from build123d import *

# Parameters (mm, degrees)
SKETCH1_R           = 17.5
BOSS_EXTRUDE1_DEPTH = 14
SKETCH2_R           = 1.5
BOSS_EXTRUDE2_DEPTH = 1
SKETCH3_R           = 5
BOSS_EXTRUDE3_DEPTH = 1.5
SKETCH4_R           = 1.5
BOSS_EXTRUDE4_DEPTH = 11
SKETCH5_R           = 3
BOSS_EXTRUDE5_DEPTH = 0.5
SKETCH6_R           = 1.5
BOSS_EXTRUDE6_DEPTH = 0.1
FILLET1_R           = 0.5
SKETCH7_W           = 7
SKETCH7_H           = 7.8
CUT_EXTRUDE3_DEPTH  = 2


with BuildPart() as part:
    # Sketch1 → Boss-Extrude1 (new body)
    with BuildSketch(Plane(origin=(0, 0, 0), x_dir=(1, 0, 0), z_dir=(0, 1, 0))):
        Circle(SKETCH1_R)
    extrude(amount=BOSS_EXTRUDE1_DEPTH)

    # Sketch2 → Boss-Extrude2 (add)
    with BuildSketch(Plane.XZ):
        with BuildLine():
            Line((14.671631406, 18.344732976), (-0.891940662, 17.553925067))
            ThreePointArc((-0.891940662, 17.553925067), (-12.428512449, 12.428512449), (-17.553925067, 0.891940662))
            Line((-17.553925067, 0.891940662), (-18.344732976, -14.671631406))
            ThreePointArc((-18.344732976, -14.671631406), (-17.324116139, -17.324116139), (-14.671631406, -18.344732976))
            Line((-14.671631406, -18.344732976), (0.891940662, -17.553925067))
            ThreePointArc((0.891940662, -17.553925067), (12.428512449, -12.428512449), (17.553925067, -0.891940662))
            Line((17.553925067, -0.891940662), (18.344732976, 14.671631406))
            ThreePointArc((18.344732976, 14.671631406), (17.324116139, 17.324116139), (14.671631406, 18.344732976))
        make_face()
        with Locations((14.849242405, 14.849242405)):
            Circle(SKETCH2_R, mode=Mode.SUBTRACT)
        with Locations((-14.849242405, -14.849242405)):
            Circle(SKETCH2_R, mode=Mode.SUBTRACT)
    extrude(amount=BOSS_EXTRUDE2_DEPTH)

    # Sketch3 → Boss-Extrude3 (add)
    with BuildSketch(Plane.XZ.offset(1)):
        Circle(SKETCH3_R)
    extrude(amount=BOSS_EXTRUDE3_DEPTH)

    # Sketch4 → Boss-Extrude4 (add)
    with BuildSketch(Plane.XZ.offset(2.5)):
        Circle(SKETCH4_R)
    extrude(amount=BOSS_EXTRUDE4_DEPTH)

    # Sketch5 → Boss-Extrude5 (add)
    with BuildSketch(Plane(origin=(0, 14, 0), x_dir=(1, 0, 0), z_dir=(0, 1, 0))):
        Circle(SKETCH5_R)
    extrude(amount=BOSS_EXTRUDE5_DEPTH)

    # Sketch6 → Boss-Extrude6 (add)
    with BuildSketch(Plane(origin=(0, 14.5, 0), x_dir=(1, 0, 0), z_dir=(0, 1, 0))):
        Circle(SKETCH6_R)
    extrude(amount=BOSS_EXTRUDE6_DEPTH)

    # Fillet1
    fillet1_edges = [part.edges().sort_by_distance(p)[0] for p in [
        (-17.5, 14, 0),
    ]]
    fillet(fillet1_edges, radius=FILLET1_R)

    # Sketch7 → Cut-Extrude3 (cut)
    with BuildSketch(Plane.XY.offset(17.5)):
        with Locations((0, 6.75)):
            Rectangle(SKETCH7_W, SKETCH7_H)
    extrude(amount=-CUT_EXTRUDE3_DEPTH, mode=Mode.SUBTRACT)


solid = part.part
Geometry: final body of the model. Coordinates: model frame, mm. A direction names the side the tool comes from. Give positions to 0.01 mm unless a question says otherwise; leave off trailing zeros. Loops run counter-clockwise (first coordinate to the right, second up) from the corner with the lowest first, then second, coordinate; pieces in that order, holes last. Notation, with made-up numbers: M 32.25,89.25 L 43.25,89.25 A25 cw 43.25,115.25 Z; hole C -3,-16.75 d2. An arc over 180 degrees is marked long. Put each result on its own line as item: value. Start each with the question number.
1) Ray query, line 1 along Y through (x, z) = (-12.5, -13.5); line 2 along Y through (x, z) = (14, 6); line 3 along X through (y, z) = (6.5, -7.5). Return the intervals inside material, ascending.
2) Access query for faces 1 (the flat face through (-3.5, 7, 16)), 2 (the cylindrical face through (12.3, -0.493, -12.556)), 3 (the cylindrical face through (-1.5, -7.92, 0.07)). Directions: +Z, -Z, +X, -X, +Y, -Y. A direction counts if a zero-diameter tool reaches every point of the face in a straight line with its end or side. Return the directions, or none.
3) Cut plane C-C (z = 0). Output: boundary loops of the cut face in (x, y).
4) Contact query for flat-ended pins moving along their axis: pin 1 (10 mm diameter, centred on x = 3, z = -7, fed in from +Y); pin 2 (1.8 mm diameter, centred on y = 8.5, z = 16.5, fed in from +X); pin 3 (5 mm diameter, centred on x = -14.85, z = -14.85, fed in from +Y); pin 4 (12 mm diameter, centred on x = 11.5, y = -8, fed in from -Z) (3 decimals). Output: stop coordinate, or through.
5) Cut plane B-B (y = 6.75). Output: boundary loops of the cut face in (x, z), then the cut area to 3 significant figures.
6) Pull-direction query (Y, two-part tool) for faces 4 (the cylindrical face through (-14.2, -0.5, -16.2)), 5 (the flat face through (0, -13.5, 0)), 6 (the flat face through (3.5, 7, 16)); classes: pulls with the +Y half, pulls with the -Y half, needs draft (parallel to the pull), parting line crosses it, or undercut.
7) Cut plane D-D (y = 0.5). Output: boundary loops of the cut face in (x, z).
Verdict:
1. line 1: -1 to 0
1. line 2: -1 to 14
1. line 3: -15.81 to 15.81
2. face 1: +Z
2. face 2: -Z, +X, +Y, -Y
2. face 3: -Y
3. outline: M -17.6,-1 L -5,-1 L -5,-2.5 L -1.5,-2.5 L -1.5,-13.5 L 1.5,-13.5 L 1.5,-2.5 L 5,-2.5 L 5,-1 L 17.6,-1 L 17.6,0 L 17.5,0 L 17.5,13.5 A0.5 ccw 17,14 L 3,14 L 3,14.5 L 1.5,14.5 L 1.5,14.6 L -1.5,14.6 L -1.5,14.5 L -3,14.5 L -3,14 L -17,14 A0.5 ccw -17.5,13.5 L -17.5,0 L -17.6,0 Z
4. pin 1: y = 14.5
4. pin 2: x = 7.93
4. pin 3: y = 0
4. pin 4: through
5. outline: M -3.5,15.5 L -3.5,17.15 A17.5 ccw long 3.5,17.15 L 3.5,15.5 Z
5. area: 949 mm2
6. face 4: needs draft
6. face 5: pulls with the -Y half
6. face 6: undercut
7. outline: C 0,0 d35
